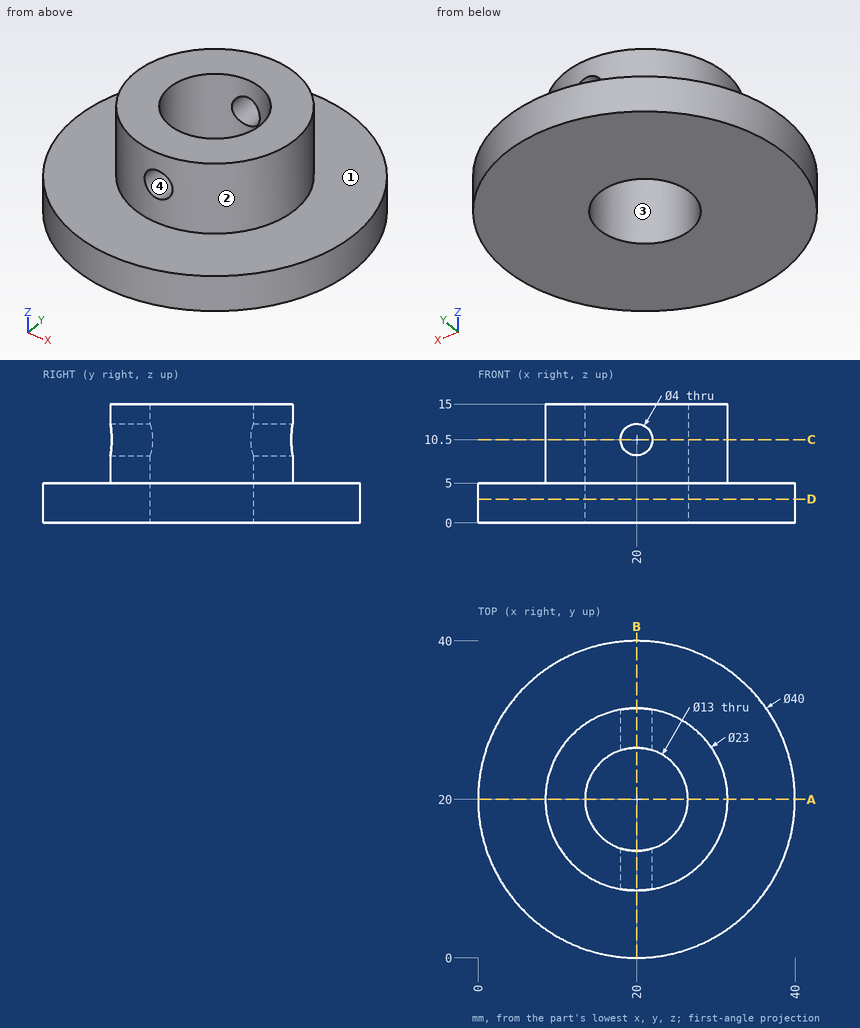
Study the drawing (mm; zero at the part's minimum x, y, z) and answer. Give positions to 0.01 mm unless a question says otherwise; leave off trailing zeros. Loops run counter-clockwise (first coordinate to the right, second up) from the corner with the lowest first, then second, coordinate; pieces in that order, holes last. Notation, with made-up numbers: M -18.5,-35.75 L 11.5,-35.75 A24 ccw 11.5,-24.75 Z; hole C -9,13.5 d2. An arc over 180 degrees is marked long. One line per item, written item: value. Start each with the question number.
1. Determine the mould class of the marked faces 1, 2, 3 and 4 for opening direction X: released by +X, released by -X, zero draft, split by the parting line, or undercut.
2. Find section A-A (y = 20). Give the vertices of the cut face in (x, z).
3. Find section C-C (z = 10.5). Give the vertices of the cut face in (x, y).
4. Find section D-D (z = 3). Give the vertices of the cut face in (x, y).
5. Each of these flat-tipped pins is pushed along its axis until it touches: P1, Ø8, axis at x = 16.5, y = 34.5, coming from the +Z side; P2, Ø2, axis at y = 29, z = 8, coming from the +X side; P3, Ø1.5, axis at x = 29.5, z = 11, coming from the -Y side; P4, Ø3, axis at x = 5, z = 7.5, coming from the -Y side. Where does it stop, or does it pass through?
6. Find section B-B (x = 20). Give the vertices of the cut face in (y, z).
7. Find the intervals of material crossed by probe 1 along Z at (x, y) = (20, 10.7); probe 2 along Y at (x, z) = (20, 5.25); probe 3 along Z at (x, y) = (36, 9), in increasing order.
Reported:
1. face 1: zero draft
1. face 2: split by the parting line
1. face 3: undercut
1. face 4: undercut
2. outline: M 0,0 L 13.5,0 L 13.5,15 L 8.5,15 L 8.5,5 L 0,5 Z; M 26.5,0 L 40,0 L 40,5 L 31.5,5 L 31.5,15 L 26.5,15 Z
3. outline: M 18,8.68 L 18,13.82 A6.5 cw 18,26.18 L 18,31.32 A11.5 ccw Z; M 22,8.68 A11.5 ccw 22,31.32 L 22,26.18 A6.5 cw 22,13.82 Z
4. outline: C 20,20 d40; hole C 20,20 d13
5. P1: stops at z = 15
5. P2: stops at x = 28.26
5. P3: stops at y = 12.54
5. P4: passes through
6. outline: M 0,0 L 13.5,0 L 13.5,8.5 L 8.5,8.5 L 8.5,5 L 0,5 Z; M 8.5,12.5 L 13.5,12.5 L 13.5,15 L 8.5,15 Z; M 26.5,0 L 40,0 L 40,5 L 31.5,5 L 31.5,8.5 L 26.5,8.5 Z; M 26.5,12.5 L 31.5,12.5 L 31.5,15 L 26.5,15 Z
7. probe 1: z = 0 to 8.5, 12.5 to 15
7. probe 2: y = 8.5 to 13.5, 26.5 to 31.5
7. probe 3: z = 0 to 5
